from build123d import *

# Parameters (mm, degrees)
SKETCH1_W           = 685
SKETCH1_H           = 250
BASE_FLANGE1_DEPTH  = 8
SKETCH6_W           = 60
SKETCH6_H           = 8
SKETCH6_W_2         = 70
EXTRUDE1_DEPTH      = 8
SKETCH7_W           = 250
SKETCH7_H           = 73.5
BASE_FLANGE2_DEPTH  = 8
SKETCH12_W          = 30.5
SKETCH12_H          = 8.5
EXTRUDE2_DEPTH      = 699.681794525
SKETCH14_W          = 250
SKETCH14_H          = 8
BASE_FLANGE3_DEPTH  = 50.5
SKETCH19_W          = 60
SKETCH19_H          = 8
SKETCH19_W_2        = 70
EXTRUDE3_DEPTH      = 8
BREAK_CORNER1_START = 41.5
BREAK_CORNER1_DEPTH = 8
EXTRUDE4_DEPTH      = 8
BASE_FLANGE4_DEPTH  = 8
SKETCH38_W          = 8.5
SKETCH38_H          = 20.5
EXTRUDE5_DEPTH      = 10
SKETCH39_W          = 20.5
SKETCH39_H          = 8.5
EXTRUDE6_DEPTH      = 10


# Read off the part's stored shape, not the designer's step: Break-Corner1
# Sheet-metal steps are written as plain solids
with BuildPart() as part:
    # Sketch1 → Base-Flange1 (new body)
    with BuildSketch(Plane(origin=(0, 0, 0), x_dir=(1, 0, 0), z_dir=(0, 1, 0))):
        Rectangle(SKETCH1_W, SKETCH1_H)
    extrude(amount=-BASE_FLANGE1_DEPTH)

    # Sketch6 → Extrude1 (cut)
    with BuildSketch(Plane(origin=(342.5, 0, 0), x_dir=(0, 0, -1), z_dir=(1, 0, 0))):
        with Locations((-95, -4)):
            Rectangle(SKETCH6_W, SKETCH6_H)
        with Locations((95, -4)):
            Rectangle(SKETCH6_W, SKETCH6_H)
        with Locations((0, -4)):
            Rectangle(SKETCH6_W_2, SKETCH6_H)
    extrude1 = extrude(amount=-EXTRUDE1_DEPTH, mode=Mode.SUBTRACT)

    # Mirror1: Extrude1 across plane
    add(extrude1.mirror(Plane(origin=(0, 0, 0), x_dir=(0, 0, 1), z_dir=(1, 0, 0))), mode=Mode.SUBTRACT)

    # Sketch39 → Extrude6 (cut)
    with BuildSketch(Plane.XZ.offset(8)):
        with Locations((289.5, 0)):
            Rectangle(SKETCH39_W, SKETCH39_H)
        with Locations((229.5, 0)):
            Rectangle(SKETCH39_W, SKETCH39_H)
        with Locations((-289.5, 0)):
            Rectangle(SKETCH39_W, SKETCH39_H)
        with Locations((-229.5, 0)):
            Rectangle(SKETCH39_W, SKETCH39_H)
    extrude(amount=-EXTRUDE6_DEPTH, mode=Mode.SUBTRACT)


with BuildPart() as body_2:
    # Sketch7 → Base-Flange2 (new body)
    with BuildSketch(Plane(origin=(334.5, 0, 0), x_dir=(0, 0, -1), z_dir=(1, 0, 0))):
        with Locations((0, 20.75)):
            Rectangle(SKETCH7_W, SKETCH7_H)
    extrude(amount=BASE_FLANGE2_DEPTH)

    # Sketch12 → Extrude2 (cut, through all)
    with BuildSketch(Plane(origin=(342.5, 0, 0), x_dir=(0, 0, -1), z_dir=(1, 0, 0))):
        with Locations((-50, -4)):
            Rectangle(SKETCH12_W, SKETCH12_H)
        with Locations((50, -4)):
            Rectangle(SKETCH12_W, SKETCH12_H)
        with Locations((50, 45.5)):
            Rectangle(SKETCH12_W, SKETCH12_H)
        with Locations((-50, 45.5)):
            Rectangle(SKETCH12_W, SKETCH12_H)
    extrude(amount=-EXTRUDE2_DEPTH, mode=Mode.SUBTRACT)

    # Sketch38 → Extrude5 (cut)
    with BuildSketch(Plane(origin=(342.5, 0, 0), x_dir=(0, 0, -1), z_dir=(1, 0, 0))):
        with Locations((0, 27.5)):
            Rectangle(SKETCH38_W, SKETCH38_H)
    extrude(amount=-EXTRUDE5_DEPTH, mode=Mode.SUBTRACT)


with BuildPart() as body_3:
    # Sketch14 → Base-Flange3 (new body)
    with BuildSketch(Plane.ZY.offset(-334.5)):
        with Locations((0, 45.5)):
            Rectangle(SKETCH14_W, SKETCH14_H)
    extrude(amount=-BASE_FLANGE3_DEPTH)

    # Sketch19 → Extrude3 (cut)
    with BuildSketch(Plane(origin=(342.5, 0, 0), x_dir=(0, 0, -1), z_dir=(1, 0, 0))):
        with Locations((95, 45.5)):
            Rectangle(SKETCH19_W, SKETCH19_H)
        with Locations((0, 45.5)):
            Rectangle(SKETCH19_W_2, SKETCH19_H)
        with Locations((-95, 45.5)):
            Rectangle(SKETCH19_W, SKETCH19_H)
    extrude(amount=-EXTRUDE3_DEPTH, mode=Mode.SUBTRACT)

    # Break-Corner1 outline → Break-Corner1 (cut)
    with BuildSketch(Plane(origin=(0, 0, 0), x_dir=(1, 0, 0), z_dir=(0, 1, 0)).offset(BREAK_CORNER1_START)):
        Polygon((385, -125), (385, -110), (370, -125), align=None)
        Polygon((370, 125), (385, 110), (385, 125), align=None)
    extrude(amount=BREAK_CORNER1_DEPTH, mode=Mode.SUBTRACT)

    # Sketch20 → Extrude4 (cut)
    with BuildSketch(Plane(origin=(0, 49.5, 0), x_dir=(1, 0, 0), z_dir=(0, 1, 0))):
        with BuildLine():
            Line((367, 75), (367, 55))
            ThreePointArc((367, 55), (362.5, 50.5), (358, 55))
            Line((358, 55), (358, 75))
            ThreePointArc((358, 75), (362.5, 79.5), (367, 75))
        make_face()
        with BuildLine():
            Line((367, -75), (367, -55))
            ThreePointArc((367, -55), (362.5, -50.5), (358, -55))
            Line((358, -55), (358, -75))
            ThreePointArc((358, -75), (362.5, -79.5), (367, -75))
        make_face()
    extrude(amount=-EXTRUDE4_DEPTH, mode=Mode.SUBTRACT)


with BuildPart() as body_4:
    # Mirror4: mirrored copy
    add(body_3.part.mirror(Plane(origin=(0, 0, 0), x_dir=(0, 0, 1), z_dir=(1, 0, 0))))


with BuildPart() as body_5:
    # Sketch29 → Base-Flange4 (new body)
    with BuildSketch(Plane.XY.offset(4)):
        Polygon((219.5, 0), (219.5, -8), (239.5, -8), (239.5, 0), (279.5, 0), (279.5, -8), (299.5, -8), (299.5, 0), (334.5, 0), (334.5, 17.5), (342.5, 17.5), (342.5, 37.5), (334.5, 37.5), (334.5, 57.5), (194.5, 10), (194.5, 0), align=None)
    extrude(amount=-BASE_FLANGE4_DEPTH)


with BuildPart() as body_6:
    # Mirror5: mirrored copy
    add(body_5.part.mirror(Plane(origin=(0, 0, 0), x_dir=(0, 0, 1), z_dir=(1, 0, 0))))


with BuildPart() as body_7:
    # Mirror3: mirrored copy
    add(body_2.part.mirror(Plane(origin=(0, 0, 0), x_dir=(0, 0, 1), z_dir=(1, 0, 0))))


solid = body_4.part
Here's how the part is built. I have some questions about the finished solid (model axes, mm). A direction names the side the tool comes from. Give positions to 0.01 mm unless a question says otherwise; leave off trailing zeros. Order: outer loops, then holes, each group sorted by start corner. A loop starts at its lowest first (then second) coordinate and runs counter-clockwise, first axis right, second up. Notation, with made-up numbers: (74, -10) -> (99, -10) arc R18 ccw to (99, -2) -> close; hole circle Ø9 at (26.25, 87). An arc over 180 degrees is marked (long way). Use a Markdown table: item, result. Add a question column.
Item 1: Will these pins go through, and if not, where does the flat tip stop? pin 1 (2.5 mm diameter, centred on y = 44.5, z = -87.5, fed in from +X); pin 2 (4 mm diameter, centred on x = -336.5, y = 47, fed in from +Z); pin 3 (4 mm diameter, centred on x = -337.5, y = 47.5, fed in from -Z).
Item 2: Imagine slicing it at A-A on y = 45.5. Please give me the cut outline in (x, z), plus the area to 3 significant figures.
Item 3: I need wall thicknesses on line 1 (X direction, y = 46, z = -71.5); line 2 (X direction, y = 43.5, z = 57.5); line 3 (X direction, y = 48, z = 91). Which ranges of each line are inside material? Lowest first, please.
Item 4: Imagine slicing it at C-C on x = -374. Please give me the cut outline in (y, z).
Item 5: For faces 4 (the face through (-339, 45, -65)), 5 (the face through (-356, 45, 125)), 6 (the face through (-339, 45, 65)), 7 (the face through (-339, 45, -35)), 8 (the face through (-367, 46, -65)), which set-ups out of +Z, -Z, +X, -X, +Y, -Y let a thin tool reach every point of the face, with its end or its side?
Item 6: Imagine slicing it at B-B on x = -362.5. Please give me the cut outline in (y, z), plus the area to 3 significant figures.
Item 7: If we mould it in two halves opening along Z, with no side actions, what happens to faces 1 (the face through (-362.6, 45.6, 50.5)), 2 (the face through (-342.5, 46, -95)), 3 (the face through (-377, 45, -118))? For each: pulls with the +Z half, pulls with the -Z half, needs draft (parallel to the pull), parting line crosses it, or undercut.
Data:
| question | item | result |
|---|---|---|
| 1 | pin 1 | stops at x = -342.5 |
| 1 | pin 2 | stops at z = 65 |
| 1 | pin 3 | stops at z = -65 |
| 2 | outline | (-385, -110) -> (-370, -125) -> (-342.5, -125) -> (-342.5, -65) -> (-334.5, -65) -> (-334.5, -35) -> (-342.5, -35) -> (-342.5, 35) -> (-334.5, 35) -> (-334.5, 65) -> (-342.5, 65) -> (-342.5, 125) -> (-370, 125) -> (-385, 110) -> close; hole (-367, -75) arc R4.5 ccw to (-358, -75) -> (-358, -55) arc R4.5 ccw to (-367, -55) -> close; hole (-367, 55) arc R4.5 ccw to (-358, 55) -> (-358, 75) arc R4.5 ccw to (-367, 75) -> close |
| 2 | area | 10,400 mm² |
| 3 | line 1 | x = -385 to -367, -358 to -342.5 |
| 3 | line 2 | x = -385 to -367, -358 to -334.5 |
| 3 | line 3 | x = -385 to -342.5 |
| 4 | outline | (41.5, -121) -> (49.5, -121) -> (49.5, 121) -> (41.5, 121) -> close |
| 5 | face 4 | -Z, +X, +Y, -Y |
| 5 | face 5 | +Z, +X, -X, +Y, -Y |
| 5 | face 6 | +Z, +X, +Y, -Y |
| 5 | face 7 | +X, +Y, -Y |
| 5 | face 8 | +Y, -Y |
| 6 | outline | (41.5, -125) -> (49.5, -125) -> (49.5, -79.5) -> (41.5, -79.5) -> close; (41.5, -50.5) -> (49.5, -50.5) -> (49.5, 50.5) -> (41.5, 50.5) -> close; (41.5, 79.5) -> (49.5, 79.5) -> (49.5, 125) -> (41.5, 125) -> close |
| 6 | area | 1,540 mm² |
| 7 | face 1 | undercut |
| 7 | face 2 | needs draft |
| 7 | face 3 | pulls with the -Z half |
